Work out the finished part from the listing and answer in its coordinate system (mm). Coordinates: 2 decimals unless noted, no trailing zeros. Order: outer loops, then holes, each group sorted by start corner. A loop starts at its lowest first (then second) coordinate and runs counter-clockwise, first axis right, second up. Notation, with made-up numbers: M 2.25,-31.75 L 47.25,-31.75 A20 cw 47.25,-19.75 Z; hole C 26.25,80 d11. An arc over 180 degrees is marked long. Use a Markdown table: item, result.
from build123d import *

# Parameters (mm, degrees)
F0_W     = 25.4
F0_H     = 50.8
F1_DEPTH = 9.398
F2_D     = 4.3688


with BuildPart() as f1:
    # F0 (on Front) → F1 (new body)
    with BuildSketch(Plane.XZ):
        Rectangle(F0_W, F0_H)
    extrude(amount=-F1_DEPTH)

    # F2 (through all)
    with Locations(Plane.XZ):
        with Locations((-9.525, 22.225), (9.525, 22.225), (9.525, -22.225), (-9.525, -22.225)):
            Hole(F2_D / 2)


solid = f1.part
1. For a pull along X with two mould halves and no side action, classify faces 1 (the face through (0, 0, 0)), 2 (the face through (-12.7, 5, 0)), 3 (the face through (-10.533, 4.765, 20.287)) as +X half, -X half, draft (parallel to the pull), parting line (faces both ways), or undercut.
Answers below:
| item | result |
|---|---|
| face 1 | draft |
| face 2 | -X half |
| face 3 | undercut |
2. Section B-B on y = 6.25 is taken. Determine the outline of the cut face in (x, z) (3 decimals).
Answers below:
| item | result |
|---|---|
| outline | M -12.7,-25.4 L 12.7,-25.4 L 12.7,25.4 L -12.7,25.4 Z; hole C -9.525,-22.225 d4.369; hole C -9.525,22.225 d4.369; hole C 9.525,-22.225 d4.369; hole C 9.525,22.225 d4.369 |
3. Find the intervals of material crossed by probe 1 along X at (y, z) = (2.75, 22); probe 2 along Z at (x, y) = (10, 6.25); probe 3 along X at (y, z) = (5.75, -20.5), in increasing order.
Answers below:
| item | result |
|---|---|
| probe 1 | -12.7 to -11.7, -7.35 to 7.35, 11.7 to 12.7 |
| probe 2 | -25.4 to -24.36, -20.09 to 20.09, 24.36 to 25.4 |
| probe 3 | -12.7 to -10.87, -8.18 to 8.18, 10.87 to 12.7 |
4. A flat-ended cylindrical pin translates along its axis: P1, Ø4, axis at x = 5.5, z = -14, coming from the -Y side. Find the tip coordinate at first contact, or state that the pin passes through.
Answers below:
| item | result |
|---|---|
| P1 | y = 0 |
5. Section A-A on x = -10.5 is taken. Determine the outline of the cut face in (y, z), then the cut area to 3 significant figures.
Answers below:
| item | result |
|---|---|
| outline | M 0,-25.4 L 9.4,-25.4 L 9.4,-24.18 L 0,-24.18 Z; M 0,-20.27 L 9.4,-20.27 L 9.4,20.27 L 0,20.27 Z; M 0,24.18 L 9.4,24.18 L 9.4,25.4 L 0,25.4 Z |
| area | 404 mm² |
